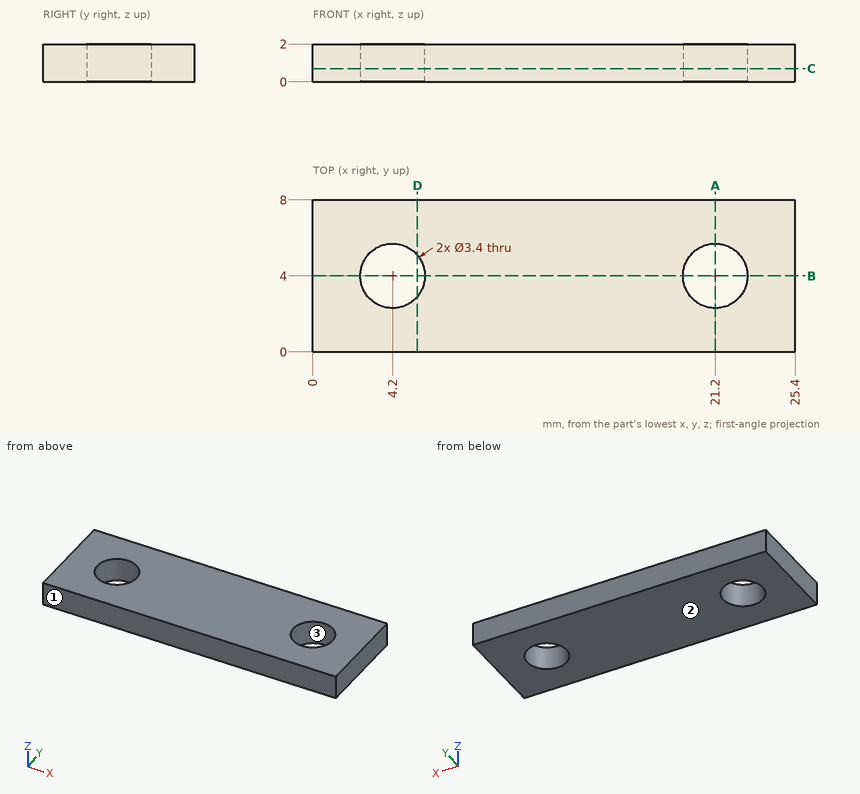
Could you check a few things on this drawing? It's one solid part, dimensions in mm from its lowest x, y, z. Give positions to 0.01 mm unless a question says otherwise; leave off trailing zeros. Order: outer loops, then holes, each group sorted by start corner. A loop starts at its lowest first (then second) coordinate and runs counter-clockwise, first axis right, second up. Notation, with made-up numbers: M 35.5,77.5 L 64.5,77.5 A5 ccw 64.5,83.5 Z; hole C 52.5,78.25 d5. An arc over 180 degrees is marked long. Use one line per item in the form item = value. Start each with the question number.
Item 1: If we section it at B-B (y = 4): Write out the boundary of the cut face in (x, z), then the cut area to 3 significant figures.
Item 2: We'd pull the mould along Y, two halves only. Please class the marked faces 1, 2 and 3: +Y half, -Y half, draft (parallel to the pull), parting line (faces both ways), or undercut.
Item 3: If I drill on line 1 along X through (y, z) = (4, 0.7); line 2 along Y through (x, z) = (4.2, 1.55); line 3 along X through (y, z) = (3.5, 1.2), over which ranges is the centre line in solid material (lowest first)?
Item 4: If we section it at D-D (x = 5.5): Write out the boundary of the cut face in (y, z), then the cut area to 3 significant figures.
Item 5: If we section it at C-C (z = 0.7): Write out the boundary of the cut face in (x, y).
Item 6: Will this pin go through, and if not, where does the flat tip stop? pin 1 Ø2 at (x, y) = (21.2, 4) entering from +Z.
Item 7: If we section it at A-A (x = 21.2): Write out the boundary of the cut face in (y, z).
Outcome:
q1.outline = M 0,0 L 2.5,0 L 2.5,2 L 0,2 Z; M 5.9,0 L 19.5,0 L 19.5,2 L 5.9,2 Z; M 22.9,0 L 25.4,0 L 25.4,2 L 22.9,2 Z
q1.area = 37.2 mm2
q2.face_1 = -Y half
q2.face_2 = draft
q2.face_3 = undercut
q3.line_1 = 0 to 2.5, 5.9 to 19.5, 22.9 to 25.4
q3.line_2 = 0 to 2.3, 5.7 to 8
q3.line_3 = 0 to 2.58, 5.82 to 19.58, 22.82 to 25.4
q4.outline = M 0,0 L 2.9,0 L 2.9,2 L 0,2 Z; M 5.1,0 L 8,0 L 8,2 L 5.1,2 Z
q4.area = 11.6 mm2
q5.outline = M 0,0 L 25.4,0 L 25.4,8 L 0,8 Z; hole C 4.2,4 d3.4; hole C 21.2,4 d3.4
q6.pin_1 = through
q7.outline = M 0,0 L 2.3,0 L 2.3,2 L 0,2 Z; M 5.7,0 L 8,0 L 8,2 L 5.7,2 Z
